Check sheet for the modelled part. Datum: model origin and axes. Units: mm. A direction names the side the tool comes from. Round coordinates to 2 decimals unless told otherwise and drop trailing zeros. Write each loop counter-clockwise with the first axis right and the second up, starting at its lowest first coordinate (ties: lowest second). Pieces come first, ordered by that corner, then holes.
Item 1: Material ranges on line 1 (Z direction, x = -91.5, y = -66); line 2 (X direction, y = -31, z = 74); line 3 (Z direction, x = -44, y = -24), recorded low to high.
Item 2: Cross-section at C-C on y = -90. Enter the section's corners in (x, z), plus the area to 3 significant figures.
Item 3: Cross-section at A-A on x = -38.5. Enter the section's corners in (y, z), plus the area to 3 significant figures.
Item 4: Tool access check on faces 1 (the flat face through (-52, -101.6, 52)), 2 (the cylindrical face through (-67.74, -49.98, 151.69)). Record the directions out of +Z, -Z, +X, -X, +Y, -Y that give a thin tool (end or side, any length) a straight path to the whole face; none if there is none.
Item 5: Go/stop test with flat-tipped pins: pin 1 Ø2 at (y, z) = (-56.5, 126.5) entering from +X; pin 2 Ø15 at (x, z) = (-30, 66.5) entering from +Y; pin 3 Ø5 at (y, z) = (-41.5, 179) entering from +X; pin 4 Ø15 at (x, y) = (-32, -38) entering from +Z. Record where each tip stops, or that it passes through.
Item 6: Cross-section at B-B on z = 91. Enter the section's corners in (x, y), plus the area to 3 significant figures.
from build123d import *

# Parameters (mm, degrees)
F0_W     = 101.6
F0_H     = 101.6
F1_DEPTH = 101.6
F2_R     = 12.7
F3_DEPTH = 101.6
F4_W     = 50.8
F4_H     = 50.8
F5_DEPTH = 50.8


with BuildPart() as f1:
    # F0 (on Front) → F1 (new body)
    with BuildSketch(Plane.XZ):
        with Locations((-50.8, 50.8)):
            Rectangle(F0_W, F0_H)
    extrude(amount=F1_DEPTH)

    # F2 (on face) → F3 (join)
    with BuildSketch(Plane.XY.offset(101.6)):
        with Locations((-58.379106, -58.563333)):
            Circle(F2_R)
    extrude(amount=F3_DEPTH)

    # F4 (on face) → F5 (cut)
    with BuildSketch(Plane.XY.offset(101.6)):
        with Locations((-25.4, -25.4)):
            Rectangle(F4_W, F4_H)
    extrude(amount=-F5_DEPTH, mode=Mode.SUBTRACT)


solid = f1.part
Response values:
1. line 1: z = 0 to 101.6
1. line 2: x = -101.6 to -50.8
1. line 3: z = 0 to 50.8
2. outline: (-101.6, 0) - (0, 0) - (0, 101.6) - (-101.6, 101.6) - close
2. area: 10,300 mm2
3. outline: (-101.6, 0) - (0, 0) - (0, 50.8) - (-50.8, 50.8) - (-50.8, 101.6) - (-101.6, 101.6) - close
3. area: 7,740 mm2
4. face 1: +Z, -Z, +X, -X, -Y
4. face 2: +Z
5. pin 1: stops at x = -45.72
5. pin 2: stops at y = -50.8
5. pin 3: passes through
5. pin 4: stops at z = 50.8
6. outline: (-101.6, -101.6) - (0, -101.6) - (0, -50.8) - (-50.8, -50.8) - (-50.8, 0) - (-101.6, 0) - close
6. area: 7,740 mm2
